Input: dimensioned drawing with shaded views. Units: mm. Origin: part minimum x, y, z. Give positions to 0.01 mm unless a question says otherwise; leave off trailing zeros. Write each loop counter-clockwise with the first axis right and the second up, starting at its lowest first coordinate (ties: lowest second). Pieces come first, ordered by that corner, then holes.
Q1. Section B-B (z = 0.3). State how many separate pieces and enclosed holes the cut face has, plus the area to 3 significant figures.
Q2. Pin query (flat end, axial travel): pin 1 Ø1.2 at (x, y) = (27.62, 11.73) entering from +Z. Return the tip coordinate at first contact, or that it passes through.
Q3. Section A-A (x = 35.24). Return the cut outline in (y, z), plus the area to 3 significant figures.
Q4. Line query: line 1 (Y direction, x = 35.24, z = 1.1); line 2 (Y direction, x = 7, z = 0.7). Output: solid intervals per line, ascending.
Q5. Section D-D (x = 12). Return the cut outline in (y, z), plus the area to 3 significant figures.
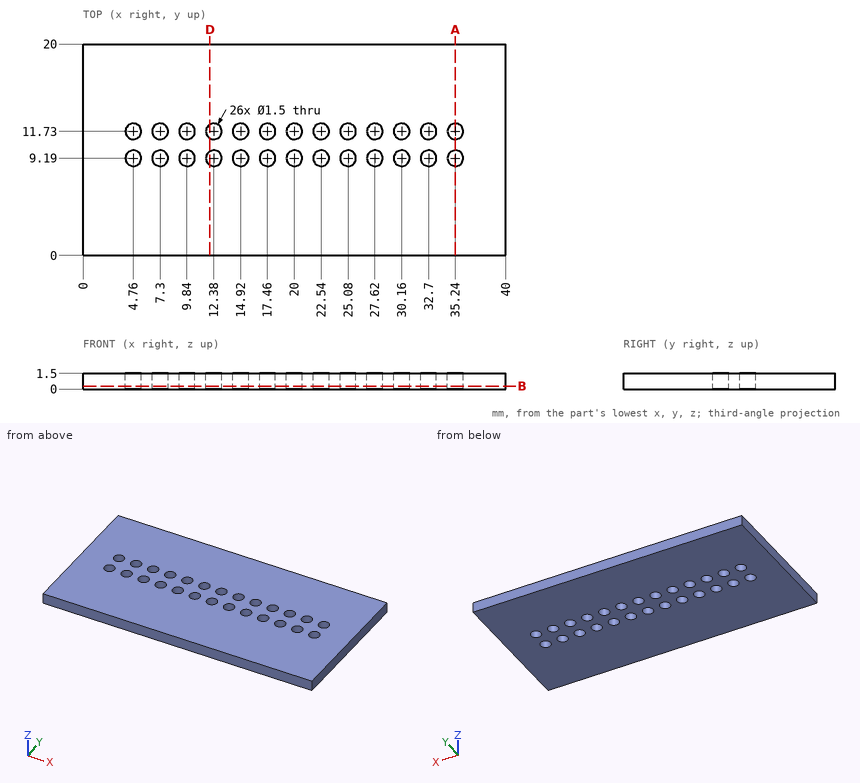
Computed:
1. separate pieces: 1
1. enclosed holes: 26
1. area: 754 mm2
2. pin 1: passes through
3. outline: (0, 0) - (8.44, 0) - (8.44, 1.5) - (0, 1.5) - close; (9.94, 0) - (10.98, 0) - (10.98, 1.5) - (9.94, 1.5) - close; (12.48, 0) - (20, 0) - (20, 1.5) - (12.48, 1.5) - close
3. area: 25.5 mm2
4. line 1: y = 0 to 8.44, 9.94 to 10.98, 12.48 to 20
4. line 2: y = 0 to 8.5, 9.88 to 11.04, 12.42 to 20
5. outline: (0, 0) - (8.54, 0) - (8.54, 1.5) - (0, 1.5) - close; (9.84, 0) - (11.08, 0) - (11.08, 1.5) - (9.84, 1.5) - close; (12.38, 0) - (20, 0) - (20, 1.5) - (12.38, 1.5) - close
5. area: 26.1 mm2
